Part print with two shaded views. Sizes in mm from the minimum x, y, z corner. A direction names the side the tool comes from. Give positions to 0.01 mm unless a question says otherwise; leave off trailing zeros. Loops run counter-clockwise (first coordinate to the right, second up) from the corner with the lowest first, then second, coordinate; pieces in that order, holes last. Notation, with made-up numbers: (43.5, -15) -> (93.5, -15) arc R27 ccw to (93.5, 4) -> close; hole circle Ø8 at (-36, -26). An arc over 180 degrees is marked (long way). One line per question, with ' | ' between items. Start each with the question number.
(1) Slice it at C-C, the plane x = 14.75. Write the cut outline in (y, z), then the cut area to 3 significant figures.
(2) Mould opens along Z. For the marked faces 3, 4 and 5 say: pulls with the +Z half, pulls with the -Z half, needs draft (parallel to the pull), parting line crosses it, or undercut.
(3) Slice it at D-D, the plane y = 2. Write the cut outline in (x, z).
(4) 3-axis set-ups, long thin cutter, end or side, ignore diameter. For the marked faces 1 and 2: which of +Z, -Z, +X, -X, +Y, -Y reach the whole face in a straight line?
(5) Slice it at B-B, the plane z = 7.75. Write the cut outline in (x, y), then the cut area to 3 significant figures.
(6) Drill centre lines: L1, parallel to Z at x = 13.75, y = 2.5; L2, parallel to X at y = 2.5, z = 17.5; L3, parallel to Y at x = 5.25, z = 3.5. Where is each one in solid material? Low to high. Write a range as from..to.
(7) Slice it at A-A, the plane z = 12.5. Write the cut outline in (x, y).
(8) Flat gauge pins, fed straight in: pin 1 Ø5 at (y, z) = (1.5, 2.5) entering from +X; pin 2 Ø4 at (x, y) = (12.5, 7) entering from -Z; pin 3 Ø5 at (y, z) = (3, 19) entering from -X; pin 4 Ø5.5 at (x, z) = (12.5, 12.5) entering from -Y. Where does each tip first touch, or does it go through?
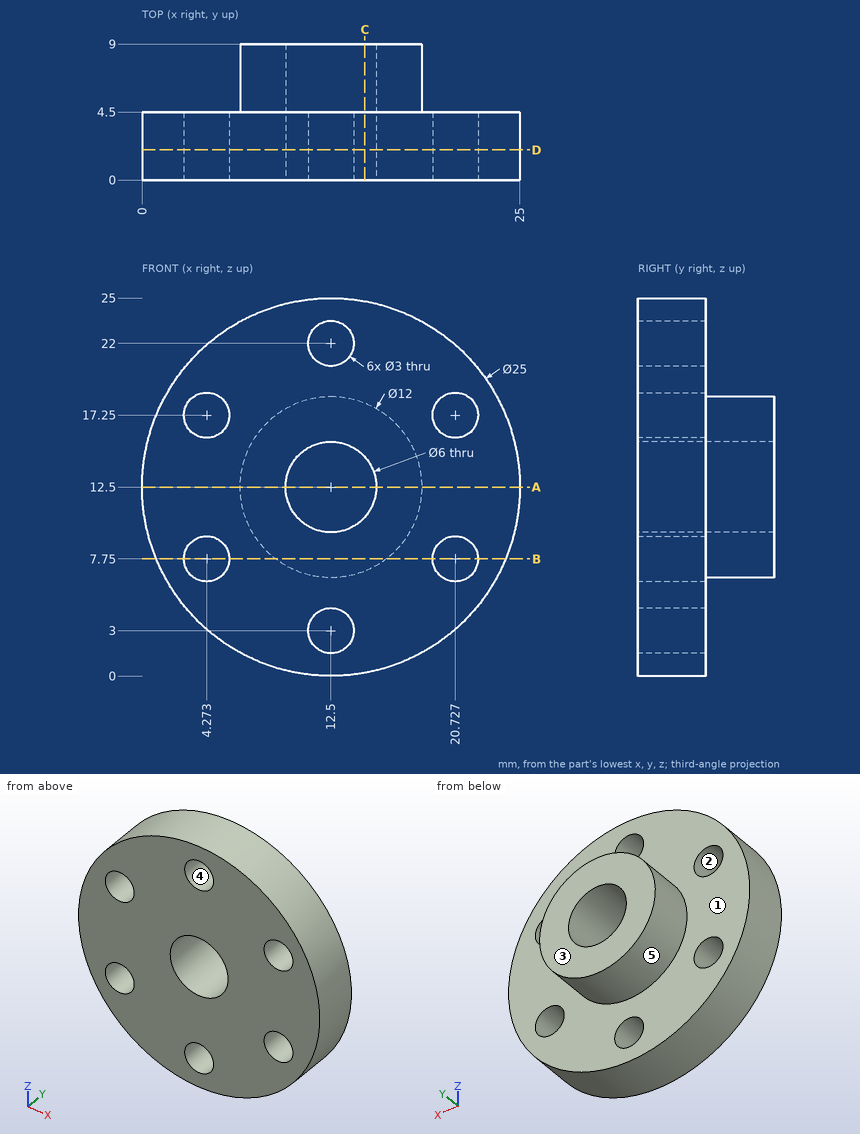
Final values:
1) outline: (0, 0.2) -> (4.5, 0.2) -> (4.5, 6.94) -> (9, 6.94) -> (9, 10.52) -> (0, 10.52) -> close; (0, 14.48) -> (9, 14.48) -> (9, 18.06) -> (4.5, 18.06) -> (4.5, 24.8) -> (0, 24.8) -> close | area: 125 mm2
2) face 3: needs draft | face 4: undercut | face 5: parting line crosses it
3) outline: circle Ø25 at (12.5, 12.5); hole circle Ø3 at (4.27, 7.75); hole circle Ø3 at (4.27, 17.25); hole circle Ø6 at (12.5, 12.5); hole circle Ø3 at (12.5, 3); hole circle Ø3 at (12.5, 22); hole circle Ø3 at (20.73, 7.75); hole circle Ø3 at (20.73, 17.25)
4) face 1: +Y | face 2: +Y, -Y
5) outline: (0.94, 0) -> (2.77, 0) -> (2.77, 4.5) -> (0.94, 4.5) -> close; (5.77, 0) -> (19.23, 0) -> (19.23, 4.5) -> (16.17, 4.5) -> (16.17, 9) -> (8.83, 9) -> (8.83, 4.5) -> (5.77, 4.5) -> close; (22.23, 0) -> (24.06, 0) -> (24.06, 4.5) -> (22.23, 4.5) -> close | area: 110 mm2
6) L1: 0.06..2.17, 3.83..9.77, 15.23..21.17, 22.83..24.94 | L2: 1.04..2.79, 5.75..19.25, 22.21..23.96 | L3: 0..4.5
7) outline: (0, 0) -> (9.5, 0) -> (9.5, 9) -> (6.5, 9) -> (6.5, 4.5) -> (0, 4.5) -> close; (15.5, 0) -> (25, 0) -> (25, 4.5) -> (18.5, 4.5) -> (18.5, 9) -> (15.5, 9) -> close
8) pin 1: x = 22.5 | pin 2: z = 6.5 | pin 3: x = 0.66 | pin 4: through
